CAD build for the part. Positions are in the model's coordinates, mm. Coordinates: 2 decimals unless noted, no trailing zeros. Order: outer loops, then holes, each group sorted by start corner. A loop starts at its lowest first (then second) coordinate and runs counter-clockwise, first axis right, second up. Notation, with made-up numbers: M 20.5,20 L 63.5,20 A16 ccw 63.5,24 Z; hole C 74.5,25.5 d3. An arc over 180 degrees is marked long. Write item = value, one per line.
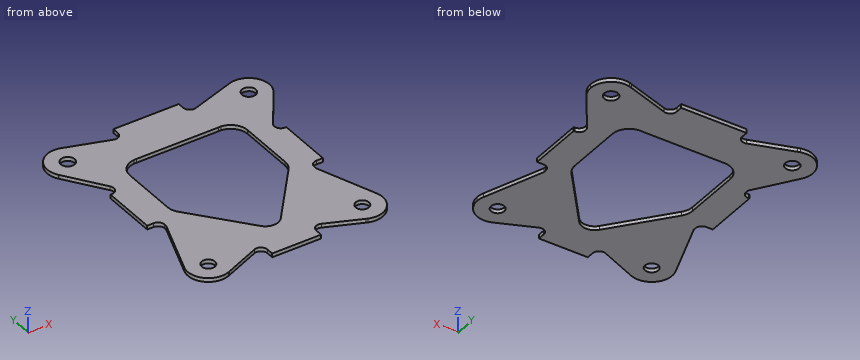
from build123d import *

# Parameters (mm, degrees)
F0_R     = 5.15
F0_R_2   = 5.35
F1_DEPTH = 3


with BuildPart() as f1:
    # F0 (on Top) → F1 (new body)
    with BuildSketch(Plane.XY):
        with BuildLine():
            Line((-18.9, -13), (0, -13))
            Line((0, -13), (18.9, -13))
            Line((18.9, -13), (18.9, -7.5471567511))
            ThreePointArc((18.9, -7.5471567511), (21.1385310794, -3.3789089897), (25.8497157602, -2.9429620925))
            Line((25.8497157602, -2.9429620925), (52.6252323996, -14.2814589745))
            ThreePointArc((52.6252323996, -14.2814589745), (48.8117732228, 11.7040295779), (74.3452534861, 5.5534627876))
            Line((74.3452534861, 5.5534627876), (57.8907951768, 50.621942028))
            Line((57.8907951768, 50.621942028), (57.8907951768, 52.621942028))
            ThreePointArc((57.8907951768, 52.621942028), (59.3552612709, 56.1574759339), (62.8907951768, 57.621942028))
            Line((62.8907951768, 57.621942028), (67.8907951768, 57.621942028))
            Line((67.8907951768, 57.621942028), (67.8907951768, 99.621942028))
            Line((67.8907951768, 99.621942028), (67.0134539994, 99.621942028))
            ThreePointArc((67.0134539994, 99.621942028), (62.5856321018, 102.2993587156), (62.8998598996, 107.4641847308))
            Line((62.8998598996, 107.4641847308), (82.9549976553, 136.4901001683))
            ThreePointArc((82.9549976553, 136.4901001683), (57.5400115252, 135.8254535138), (64.1829778441, 160.3659154829))
            Line((64.1829778441, 160.3659154829), (31.8054457349, 149.7677431215))
            ThreePointArc((31.8054457349, 149.7677431215), (27.315483743, 150.4713614419), (25.25, 154.5196467995))
            Line((25.25, 154.5196467995), (25.25, 159.621942028))
            Line((25.25, 159.621942028), (0, 159.621942028))
            Line((0, 159.621942028), (-25.25, 159.621942028))
            Line((-25.25, 159.621942028), (-25.25, 154.5196467995))
            ThreePointArc((-25.25, 154.5196467995), (-27.315483743, 150.4713614419), (-31.8054457349, 149.7677431215))
            Line((-31.8054457349, 149.7677431215), (-64.1829778441, 160.3659154829))
            ThreePointArc((-64.1829778441, 160.3659154829), (-56.8961398594, 154.5388556989), (-54.15, 145.621942028))
            ThreePointArc((-54.15, 145.621942028), (-65.2101259326, 130.5130173006), (-82.9549976553, 136.4901001683))
            Line((-82.9549976553, 136.4901001683), (-62.8998598996, 107.4641847308))
            ThreePointArc((-62.8998598996, 107.4641847308), (-62.5856321018, 102.2993587156), (-67.0134539994, 99.621942028))
            Line((-67.0134539994, 99.621942028), (-67.8907951768, 99.621942028))
            Line((-67.8907951768, 99.621942028), (-67.8907951768, 57.621942028))
            Line((-67.8907951768, 57.621942028), (-62.8907951768, 57.621942028))
            ThreePointArc((-62.8907951768, 57.621942028), (-59.3552612709, 56.1574759339), (-57.8907951768, 52.621942028))
            Line((-57.8907951768, 52.621942028), (-57.8907951768, 50.621942028))
            Line((-57.8907951768, 50.621942028), (-74.3452534861, 5.5534627876))
            ThreePointArc((-74.3452534861, 5.5534627876), (-56.6781892121, 15.5967908198), (-43.65, 0))
            ThreePointArc((-43.65, 0), (-46.0800974954, -8.4337842495), (-52.6252323996, -14.2814589745))
            Line((-52.6252323996, -14.2814589745), (-25.8497157602, -2.9429620925))
            ThreePointArc((-25.8497157602, -2.9429620925), (-21.1385310794, -3.3789089897), (-18.9, -7.5471567511))
            Line((-18.9, -7.5471567511), (-18.9, -13))
        make_face()
        with BuildLine():
            Line((-31.5007925391, 123.621942028), (0, 123.621942028))
            Line((0, 123.621942028), (31.5007925391, 123.621942028))
            ThreePointArc((31.5007925391, 123.621942028), (32.5003962696, 123.6604300644), (33.5, 123.621942028))
            ThreePointArc((33.5, 123.621942028), (42.0051009072, 119.5295106115), (45.5, 110.7619330287))
            ThreePointArc((45.5, 110.7619330287), (45.5002972018, 110.7111819333), (45.5003962696, 110.6604300644))
            ThreePointArc((45.5003962696, 110.6604300644), (45.5002972018, 110.6096781955), (45.5, 110.5589271001))
            Line((45.5, 110.5589271001), (45.5, 67.6264936436))
            ThreePointArc((45.5, 67.6264936436), (44.7475202166, 63.2677956104), (42.5771925315, 59.413687139))
            Line((42.5771925315, 59.413687139), (7.7516868511, 16.6824568887))
            Line((7.7516868511, 16.6824568887), (0, 7.1710626049))
            Line((0, 7.1710626049), (-7.7516866199, 16.6824566051))
            Line((-7.7516866199, 16.6824566051), (-42.5771925315, 59.413687139))
            ThreePointArc((-42.5771925315, 59.413687139), (-44.7475202166, 63.2677956104), (-45.5, 67.6264936436))
            Line((-45.5, 67.6264936436), (-45.5, 110.5589271001))
            ThreePointArc((-45.5, 110.5589271001), (-45.5003962696, 110.6604300644), (-45.5, 110.7619330287))
            ThreePointArc((-45.5, 110.7619330287), (-42.0051009072, 119.5295106115), (-33.5, 123.621942028))
            ThreePointArc((-33.5, 123.621942028), (-32.5003962696, 123.6604300644), (-31.5007925391, 123.621942028))
        make_face(mode=Mode.SUBTRACT)
        with BuildLine():
            ThreePointArc((74.3452534861, 5.5534627876), (48.8117732228, 11.7040295779), (52.6252323996, -14.2814589745))
            Line((52.6252323996, -14.2814589745), (54.0278478598, -14.8754176733))
            Line((54.0278478598, -14.8754176733), (74.3452534861, 5.5534627876))
        make_face()
        with Locations((59.5, 0)):
            Circle(F0_R, mode=Mode.SUBTRACT)
        with BuildLine():
            Line((54.0278478598, -14.8754176733), (52.6252323996, -14.2814589745))
            ThreePointArc((52.6252323996, -14.2814589745), (53.31940104, -14.5952970678), (54.0278478598, -14.8754176733))
        make_face()
        with BuildLine():
            Line((-54.0278478598, -14.8754176733), (-52.6252323996, -14.2814589745))
            ThreePointArc((-52.6252323996, -14.2814589745), (-46.0800974954, -8.4337842495), (-43.65, 0))
            ThreePointArc((-43.65, 0), (-56.6781892121, 15.5967908198), (-74.3452534861, 5.5534627876))
            Line((-74.3452534861, 5.5534627876), (-54.0278478598, -14.8754176733))
        make_face()
        with Locations((-59.5, 0)):
            Circle(F0_R, mode=Mode.SUBTRACT)
        with BuildLine():
            ThreePointArc((-54.0278478598, -14.8754176733), (-53.31940104, -14.5952970678), (-52.6252323996, -14.2814589745))
            Line((-52.6252323996, -14.2814589745), (-54.0278478598, -14.8754176733))
        make_face()
        with BuildLine():
            Line((74.3452534861, 5.5534627876), (54.0278478598, -14.8754176733))
            ThreePointArc((54.0278478598, -14.8754176733), (68.5688722722, -12.9991559615), (75.35, 0))
            ThreePointArc((75.35, 0), (75.0967908198, 2.8218107879), (74.3452534861, 5.5534627876))
        make_face()
        with BuildLine():
            ThreePointArc((-74.3452534861, 5.5534627876), (-70.7382626073, -11.1769384703), (-54.0278478598, -14.8754176733))
            Line((-54.0278478598, -14.8754176733), (-74.3452534861, 5.5534627876))
        make_face()
        with BuildLine():
            ThreePointArc((64.1829778441, 160.3659154829), (57.5400115252, 135.8254535138), (82.9549976553, 136.4901001683))
            Line((82.9549976553, 136.4901001683), (83.1240413462, 136.7347580678))
            Line((83.1240413462, 136.7347580678), (65.9729166922, 160.9518180885))
            Line((65.9729166922, 160.9518180885), (64.1829778441, 160.3659154829))
        make_face()
        with Locations((70, 145.621942028)):
            Circle(F0_R_2, mode=Mode.SUBTRACT)
        with BuildLine():
            Line((83.1240413462, 136.7347580678), (82.9549976553, 136.4901001683))
            ThreePointArc((82.9549976553, 136.4901001683), (83.0400932966, 136.6120326601), (83.1240413462, 136.7347580678))
        make_face()
        with BuildLine():
            Line((65.9729166922, 160.9518180885), (83.1240413462, 136.7347580678))
            ThreePointArc((83.1240413462, 136.7347580678), (85.1531936459, 140.9740153578), (85.85, 145.621942028))
            ThreePointArc((85.85, 145.621942028), (79.6797011724, 158.1728736752), (65.9729166922, 160.9518180885))
        make_face()
        with BuildLine():
            ThreePointArc((65.9729166922, 160.9518180885), (65.0692370204, 160.6854766875), (64.1829778441, 160.3659154829))
            Line((64.1829778441, 160.3659154829), (65.9729166922, 160.9518180885))
        make_face()
        with BuildLine():
            ThreePointArc((-83.1240413462, 136.7347580678), (-83.0400932966, 136.6120326601), (-82.9549976553, 136.4901001683))
            Line((-82.9549976553, 136.4901001683), (-83.1240413462, 136.7347580678))
        make_face()
        with BuildLine():
            Line((-83.1240413462, 136.7347580678), (-82.9549976553, 136.4901001683))
            ThreePointArc((-82.9549976553, 136.4901001683), (-65.2101259326, 130.5130173006), (-54.15, 145.621942028))
            ThreePointArc((-54.15, 145.621942028), (-56.8961398594, 154.5388556989), (-64.1829778441, 160.3659154829))
            Line((-64.1829778441, 160.3659154829), (-65.9729166922, 160.9518180885))
            Line((-65.9729166922, 160.9518180885), (-83.1240413462, 136.7347580678))
        make_face()
        with Locations((-70, 145.621942028)):
            Circle(F0_R_2, mode=Mode.SUBTRACT)
        with BuildLine():
            ThreePointArc((-65.9729166922, 160.9518180885), (-82.9346496049, 154.7825828134), (-83.1240413462, 136.7347580678))
            Line((-83.1240413462, 136.7347580678), (-65.9729166922, 160.9518180885))
        make_face()
        with BuildLine():
            ThreePointArc((-64.1829778441, 160.3659154829), (-65.0692370204, 160.6854766875), (-65.9729166922, 160.9518180885))
            Line((-65.9729166922, 160.9518180885), (-64.1829778441, 160.3659154829))
        make_face()
        with BuildLine():
            Line((0, 7.1710626049), (7.7516868511, 16.6824568887))
            ThreePointArc((7.7516868511, 16.6824568887), (1.829e-07, 13), (-7.7516866199, 16.6824566051))
            Line((-7.7516866199, 16.6824566051), (0, 7.1710626049))
        make_face()
    extrude(amount=F1_DEPTH)


solid = f1.part
(1) Slice it at C-C, the plane x = 70. Write the cut outline in (y, z).
Evaluation:
outline = M -11.87,0 L 17.46,0 L 17.46,3 L -11.87,3 Z; M 117.74,0 L 140.27,0 L 140.27,3 L 117.74,3 Z; M 150.97,0 L 161.47,0 L 161.47,3 L 150.97,3 Z
(2) Wall check: line 1 (X direction, y = 3, z = 2.5); line 2 (X direction, y = 110, z = 2.25); line 3 (X direction, y = 136.5, z = 0.4). Give the ranges that are in metal, low to high. Write a range as from..to.
Evaluation:
line_1 = -75.06..-63.69, -55.31..55.31, 63.69..75.06
line_2 = -64.65..-45.5, 45.5..64.65
line_3 = -82.96..82.96
(3) Slice it at B-B, the plane x = 35.5. Write the cut outline in (y, z).
Evaluation:
outline = M -7.03,0 L 50.73,0 L 50.73,3 L -7.03,3 Z; M 123.31,0 L 150.98,0 L 150.98,3 L 123.31,3 Z
(4) Slice it at A-A, the plane y = 76.5. Write the cut outline in (x, z), then the cut area to 3 significant figures.
Evaluation:
outline = M -67.89,0 L -45.5,0 L -45.5,3 L -67.89,3 Z; M 45.5,0 L 67.89,0 L 67.89,3 L 45.5,3 Z
area = 134 mm²
(5) Slice it at D-D, the plane z = 1.3. State how many separate pieces and enclosed holes the cut face has, then the cut area to 3 significant figures.
Evaluation:
separate_pieces = 1
enclosed_holes = 5
area = 15,400 mm²
(6) Pin check, flat tips, straight feed: pin 1 Ø1.5 at (y, z) = (156, 2) entering from +X; pin 2 Ø9.5 at (x, y) = (59.5, 0) entering from +Z; pin 3 Ø1.6 at (y, z) = (52, 2) entering from -X; pin 4 Ø1 at (x, z) = (-67.5, 1) entering from +Y. Stop position of each tip, or through.
Evaluation:
pin_1 = 82.59
pin_2 = through
pin_3 = -57.89
pin_4 = 161.35
